For this review, take the finished solid that the model builds, in its own axes (mm). Coordinates: 2 decimals unless noted, no trailing zeros. Loops run counter-clockwise (first coordinate to the right, second up) from the corner with the lowest first, then second, coordinate; pieces in that order, holes last. Notation, with made-up numbers: M -34.75,85 L 4.25,85 A37 ccw 4.25,123 Z; hole C 47,1.5 d9. An arc over 180 degrees is marked long. Put each result on its own line as item: value.
Autodesk Inventor part; units mm, degrees
ref_plane "YZ Plane" through (0, 0, 0) normal (1, 0, 0) x (0, 1, 0)
ref_plane "XZ Plane" through (0, 0, 0) normal (0, 1, 0) x (-1, 0, 0)
ref_plane "XY Plane" through (0, 0, 0) normal (0, 0, 1) x (1, 0, 0)
sketch "Sketch1" plane through (0, 0, 0) normal (0, 0, 1) x (1, 0, 0)
  line L0 (0, 0) -> (28, 0)
  line L1 (28, 0) -> (28, 43.4)
  line L2 (28, 43.4) -> (0, 43.4)
  line L3 (0, 43.4) -> (0, 0)
  line L4 (2.5, 40.9) -> (25.5, 40.9) construction
  line L5 (25.5, 40.9) -> (25.5, 2.5) construction
  line L6 (25.5, 2.5) -> (2.5, 2.5) construction
  line L7 (2.5, 2.5) -> (2.5, 40.9) construction
  circle A0 centre (2.5, 40.9) radius 1.5
  circle A1 centre (25.5, 40.9) radius 1.5
  circle A2 centre (25.5, 2.5) radius 1.5
  circle A3 centre (2.5, 2.5) radius 1.5
  dimension "d0" = 28
  dimension "d1" = 43.4
  dimension "d2" = 2.5
  dimension "d3" = 3
  dimension "d4" = 3
  dimension "d5" = 3
  dimension "d6" = 3
extrude "Extrusion1" add sketch "Sketch1" along normal blind 5
properties part number "GA010" material "ABS Plastic"
(1) Add section B-B (x = 25.5). Write out the cut boundary in (y, z).
Determined:
outline: M 0,0 L 1,0 L 1,5 L 0,5 Z; M 4,0 L 39.4,0 L 39.4,5 L 4,5 Z; M 42.4,0 L 43.4,0 L 43.4,5 L 42.4,5 Z
(2) For pin 1 (1.8 mm diameter, centred on x = 2.5, y = 2.5, fed in from -Z); pin 2 (1 mm diameter, centred on x = 25, z = 2, fed in from -Y), all flat-tipped, find the tip position at first contact; note any pin that passes through.
Determined:
pin 1: passes through
pin 2: stops at y = 0
(3) Add section C-C (y = 40.9). Write out the cut boundary in (x, z), plus the area to 3 significant figures.
Determined:
outline: M 0,0 L 1,0 L 1,5 L 0,5 Z; M 4,0 L 24,0 L 24,5 L 4,5 Z; M 27,0 L 28,0 L 28,5 L 27,5 Z
area: 110 mm^2
(4) Add section A-A (z = 3.2). Write out the cut boundary in (x, y).
Determined:
outline: M 0,0 L 28,0 L 28,43.4 L 0,43.4 Z; hole C 2.5,2.5 d3; hole C 2.5,40.9 d3; hole C 25.5,2.5 d3; hole C 25.5,40.9 d3
(5) Draft analysis for pull direction Y (two halves, no side actions). For faces 1 (the cylindrical face through (24, 2.43, 2.46)), 2 (the cylindrical face through (2.305, 1.013, 2.465)), 3 (the flat face through (14, 43.4, 2)), 4 (the flat face through (28, 21, 2)), state which applies: +Y half, -Y half, draft (parallel to the pull), parting line (faces both ways), or undercut.
Determined:
face 1: undercut
face 2: undercut
face 3: +Y half
face 4: draft
(6) Wall thickness on line 1 along Y through (x, z) = (25.5, 3.7); line 2 along X through (y, z) = (2, 2.25): over which ranges is each line inside the solid? List them lowest first. Write a range as [from, to].
Determined:
line 1: y = [0, 1], [4, 39.4], [42.4, 43.4]
line 2: x = [0, 1.09], [3.91, 24.09], [26.91, 28]
